Part model, mm, in its own coordinate system. A direction names the side the tool comes from. Coordinates: 2 decimals unless noted, no trailing zeros. Write each loop counter-clockwise with the first axis right and the second up, starting at its lowest first coordinate (ties: lowest second). Pieces come first, ordered by that corner, then holes. Notation, with made-up numbers: M 29.5,80.5 L 69.5,80.5 A23 ccw 69.5,99.5 Z; hole C -12.75,21 d6. An arc over 180 degrees is marked long. Use a Markdown table: item, result. Add a question column.
Q1. Slice it at C-C on y = 4.5. Write the cut outline in (x, z), then the cut area to 3 significant figures.
Q2. Pin check, flat tips, straight feed: pin 1 Ø2 at (x, y) = (-13, -13) entering from +Z; pin 2 Ø1.5 at (x, z) = (0.5, 13.5) entering from +Y; pin 3 Ø3 at (x, z) = (-8.5, 3) entering from +Y; pin 4 Ø17.5 at (x, y) = (-4, 5) entering from +Z. Stop position of each tip, or through.
Q3. Tool access for faces 1 (the flat face through (-16, 16, -18)), 2 (the cylindrical face through (-12.84, 14.24, -2.54)): list every direction of +Z, -Z, +X, -X, +Y, -Y with a clear straight run to the whole face (end or side of a thin tool).
Q4. Slice it at D-D on z = 14. Write the cut outline in (x, y).
Q5. Slice it at B-B on x = 0. Write the cut outline in (y, z).
Q6. Slice it at A-A on z = -2.5. Write the cut outline in (x, y).
Q7. Mould opens along X. For faces 3 (the flat face through (-8, 8, 0)), 4 (the cylindrical face through (0.1, -2.5, 11.4)), 5 (the flat face through (-17.5, 0, -18)), 6 (the conical face through (12.84, 13.15, -5.62)) say: released by +X, released by -X, zero draft, split by the parting line, or undercut.
Q8. Wall check: L1, parallel to Y at x = 13, z = -3.55; L2, parallel to Z at x = -5.5, y = 11.5. Give the ranges that are in metal, low to high. Write a range as from..to.
from build123d import *

# Parameters (mm, degrees)
BOSS_EXTRUDE1_DEPTH       = 36
SKETCH1_3_R               = 11
BOSS_EXTRUDE2_DEPTH       = 2
M3X0_5_TAPPED_HOLE1_D     = 2.5
M3X0_5_TAPPED_HOLE1_DEPTH = 5
M3X0_5_TAPPED_HOLE1_TIP   = 0.751075774
BOSS_EXTRUDE3_DEPTH       = 21


with BuildPart() as part:
    # Sketch1 → Boss-Extrude1 (new body)
    with BuildSketch(Plane.XY):
        Polygon((-14.5, 17.5), (-17.5, 14.5), (-17.5, -14.5), (-14.5, -17.5), (14.5, -17.5), (17.5, -14.5), (17.5, 14.5), (14.5, 17.5), align=None)
    extrude(amount=-BOSS_EXTRUDE1_DEPTH)

    # Sketch1_3 → Boss-Extrude2 (add)
    with BuildSketch(Plane.XY):
        Circle(SKETCH1_3_R)
    extrude(amount=BOSS_EXTRUDE2_DEPTH)

    # M3x0.5 Tapped Hole1
    with Locations(Plane.XY):
        with Locations((13, 13), (-13, 13), (-13, -13), (13, -13)):
            Hole(M3X0_5_TAPPED_HOLE1_D / 2, depth=M3X0_5_TAPPED_HOLE1_DEPTH)
            with Locations((0, 0, -(M3X0_5_TAPPED_HOLE1_DEPTH + M3X0_5_TAPPED_HOLE1_TIP / 2))):  # 118° drill point
                Cone(0, M3X0_5_TAPPED_HOLE1_D / 2, M3X0_5_TAPPED_HOLE1_TIP, mode=Mode.SUBTRACT)

    # Sketch1_4 → Boss-Extrude3 (add)
    with BuildSketch(Plane.XY):
        with BuildLine():
            Line((-1.5, 2), (1.5, 2))
            ThreePointArc((1.5, 2), (0, -2.5), (-1.5, 2))
        make_face()
    extrude(amount=BOSS_EXTRUDE3_DEPTH)


solid = part.part
Recorded:
| question | item | result |
|---|---|---|
| 1 | outline | M -17.5,-36 L 17.5,-36 L 17.5,0 L 10.04,0 L 10.04,2 L -10.04,2 L -10.04,0 L -17.5,0 Z |
| 1 | area | 1,300 mm² |
| 2 | pin 1 | z = -5.15 |
| 2 | pin 2 | y = 2 |
| 2 | pin 3 | y = 8.16 |
| 2 | pin 4 | z = 21 |
| 3 | face 1 | +Z, -Z, -X, +Y |
| 3 | face 2 | +Z |
| 4 | outline | M -1.5,2 A2.5 ccw long 1.5,2 Z |
| 5 | outline | M -17.5,-36 L 17.5,-36 L 17.5,0 L 11,0 L 11,2 L 2,2 L 2,21 L -2.5,21 L -2.5,2 L -11,2 L -11,0 L -17.5,0 Z |
| 6 | outline | M -17.5,-14.5 L -14.5,-17.5 L 14.5,-17.5 L 17.5,-14.5 L 17.5,14.5 L 14.5,17.5 L -14.5,17.5 L -17.5,14.5 Z; hole C -13,-13 d2.5; hole C -13,13 d2.5; hole C 13,-13 d2.5; hole C 13,13 d2.5 |
| 7 | face 3 | zero draft |
| 7 | face 4 | split by the parting line |
| 7 | face 5 | released by -X |
| 7 | face 6 | undercut |
| 8 | L1 | -17.5..-14.25, -11.75..11.75, 14.25..17.5 |
| 8 | L2 | -36..0 |
